```python
from build123d import *

# Parameters (mm, degrees)
SKETCH2_R               = 22.5
BOSS_EXTRUDE1_DEPTH     = 15
BOSS_EXTRUDE2_DEPTH     = 22
CUT_EXTRUDE2_DEPTH      = 119.676029593
CUT_EXTRUDE2_DEPTH_BACK = 119.676029593
FILLET1_R               = 100
CUT_EXTRUDE3_START      = -27.5
CUT_EXTRUDE3_DEPTH      = 4
CUT_EXTRUDE3_DRAFT      = -3
CUT_EXTRUDE7_DEPTH      = 183.208671748
CUT_EXTRUDE7_DEPTH_BACK = 183.208671748


with BuildPart() as part:
    # Sketch2 → Boss-Extrude1 (new body)
    with BuildSketch(Plane(origin=(0, 0, 0), x_dir=(0, 0, -1), z_dir=(1, 0, 0))):
        Circle(SKETCH2_R)
    extrude(amount=BOSS_EXTRUDE1_DEPTH)

    # Sketch3 → Boss-Extrude2 (add)
    with BuildSketch(Plane(origin=(0, 0, 0), x_dir=(0, 0, -1), z_dir=(1, 0, 0))):
        with BuildLine():
            Line((-27.5, 0), (-27.5, -20))
            Line((-27.5, -20), (-60, -40))
            ThreePointArc((-60, -40), (0, -100), (60, -40))
            Line((60, -40), (27.5, -20))
            Line((27.5, -20), (27.5, 0))
            ThreePointArc((27.5, 0), (0, 27.5), (-27.5, 0))
        make_face()
    extrude(amount=-BOSS_EXTRUDE2_DEPTH)

    # Sketch4 → Cut-Extrude2 (cut, two sides: drawn at the far end of the back side and taken through both)
    with BuildSketch(Plane.XY.offset(-CUT_EXTRUDE2_DEPTH_BACK)):
        Polygon((-12, 27.5), (-22, 27.5), (-22, -62.5), align=None)
    extrude(amount=CUT_EXTRUDE2_DEPTH + CUT_EXTRUDE2_DEPTH_BACK, mode=Mode.SUBTRACT)

    # Fillet1
    fillet1_edges = [part.edges().sort_by_distance(p)[0] for p in [
        (-22, -62.5, 0),
    ]]
    fillet(fillet1_edges, radius=FILLET1_R)

    # Sketch6 → Revolve1 (revolve)
    with BuildSketch(Plane.XY, mode=Mode.PRIVATE) as revolve1_sk:
        Polygon((-17, -17.5), (-45, -17.5), (-45, -25), (-60, -25), (-60, -27.5), (-110, -27.5), (-110, -40), (-17, -40), align=None)
    revolve(revolve1_sk.sketch.rotate(Axis((0, -40, 0), (1, 0, 0)), 90), axis=Axis((0, -40, 0), (1, 0, 0)))


with BuildPart() as cut_extrude3_tool:
    # Sketch8 → Cut-Extrude3 (with draft: the straight prism first)
    with BuildSketch(Plane(origin=(0, 0, 0), x_dir=(1, 0, 0), z_dir=(0, 1, 0)).offset(CUT_EXTRUDE3_START)):
        with BuildLine():
            ThreePointArc((-82, -4), (-78, 0), (-82, 4))
            Line((-82, 4), (-102, 4))
            ThreePointArc((-102, 4), (-106, 0), (-102, -4))
            Line((-102, -4), (-82, -4))
        make_face()
    extrude(amount=-CUT_EXTRUDE3_DEPTH)
    # Cut-Extrude3: the draft: its side faces are tilted about the plane it starts from
    cut_extrude3_sides = [cut_extrude3_tool.faces().sort_by_distance(p)[0] for p in [
        (-78, -29.5, 0),
        (-92, -29.5, -4),
        (-106, -29.5, 0),
        (-92, -29.5, 4),
    ]]
    draft(cut_extrude3_sides, Plane(origin=(0, 0, 0), x_dir=(1, 0, 0), z_dir=(0, 1, 0)).offset(CUT_EXTRUDE3_START), CUT_EXTRUDE3_DRAFT)


with BuildPart() as part_1:
    add(part.part)

    # Cut-Extrude3: cut by cut_extrude3_tool
    add(cut_extrude3_tool.part, mode=Mode.SUBTRACT)

    # Mirror2: part across plane


with BuildPart() as part_2:
    add(part_1.part)
    add(part_1.part.mirror(Plane(origin=(15, 0, 0), x_dir=(0, 0, 1), z_dir=(1, 0, 0))))

    # Sketch9 → Cut-Extrude7 (cut, two sides: drawn at the far end of the back side and taken through both)
    with BuildSketch(Plane.XY.offset(-CUT_EXTRUDE7_DEPTH_BACK)):
        Polygon((-60, -63.744180842), (-60, 19.972023277), (-60, 24.234333035), (-120.234198747, 24.234333035), (-120.234198747, -63.744180842), align=None)
    extrude(amount=CUT_EXTRUDE7_DEPTH + CUT_EXTRUDE7_DEPTH_BACK, mode=Mode.SUBTRACT)


solid = part_2.part
```
CAD build for the part. Positions are in the model's coordinates, mm. A direction names the side the tool comes from. Round coordinates to 2 decimals unless told otherwise and drop trailing zeros. Loops run counter-clockwise (first coordinate to the right, second up) from the corner with the lowest first, then second, coordinate; pieces in that order, holes last. Notation, with made-up numbers: M 5,37 L 57,37 A37 ccw 57,76 Z; hole C 0.5,10.25 d7. An arc over 180 degrees is marked long. Return JSON: item names as keys, results as strings. Group by question number.
(1) Saw through at D-D, the plane y = -50. List the corners of the cut face in (x, z).
(2) Tool access for faces 1 (the flat face through (-9, -10, 27.5)), 2 (the flat face through (-9, -10, -27.5)), 3 (the cylindrical face through (-31.196, -18.035, -4.878)): list every direction of +Z, -Z, +X, -X, +Y, -Y with a clear straight run to the whole face (end or side of a thin tool).
(3) Drop flat-ended pins along their axis: P1, Ø12, axis at y = -58, z = 32.5, coming from the +X side; P2, Ø16, axis at y = -83.5, z = -25, coming from the -X side; P3, Ø8, axis at x = -4.5, z = 46, coming from the -Y side. Give the stop position or say it passes through.
(4) Saw through at B-B, the plane x = -7.5. List the corners of the cut face in (y, z), and give its area (3 significant figures).
(5) Mould opens along X. For faces 4 (the conical face through (135.896, -29.472, -0.086)), 5 (the flat face through (39.61, -29.86, 43.52)), 6 (the flat face through (75, -35, 15)) say: +X half, -X half, draft (parallel to the pull), parting line (faces both ways), or undercut.
(6) Wall check: probe 1 along X at (y, z) = (-73, -39); probe 2 along X at (y, z) = (-29, -1); probe 3 along X at (y, z) = (0, -27). Give the ranges that are in metal, low to high. Write a range as [from, to].
(7) Saw through at A-A, the plane y = -88. List the corners of the cut face in (x, z), and give its area (3 significant figures).
Answer list:
{
 "1": {"outline": "M -60,-11.18 L -45,-11.18 L -45,-20.16 L -20.61,-20.16 L -20.61,-59.16 L 0,-59.16 L 0,59.16 L -20.61,59.16 L -20.61,20.16 L -45,20.16 L -45,11.18 L -60,11.18 Z; M 30,-59.16 L 50.61,-59.16 L 50.61,-20.16 L 75,-20.16 L 75,-11.18 L 90,-11.18 L 90,-7.5 L 140,-7.5 L 140,7.5 L 90,7.5 L 90,11.18 L 75,11.18 L 75,20.16 L 50.61,20.16 L 50.61,59.16 L 30,59.16 Z"},
 "2": {"face 1": "+Z, +X, -X, +Y", "face 2": "-Z, +X, -X, +Y", "face 3": "-X"},
 "3": {"P1": "x = 51.92", "P2": "x = -22", "P3": "y = -82.85"},
 "4": {"outline": "M -40,-60 L -20,-27.5 L 0,-27.5 A27.5 ccw 0,27.5 L -20,27.5 L -40,60 A60 ccw Z", "area": "9,690 mm2"},
 "5": {"face 4": "undercut", "face 5": "draft", "face 6": "+X half"},
 "6": {"probe 1": "[-22, 0], [30, 52]", "probe 2": "[-60, 0], [30, 108.21], [135.79, 140]", "probe 3": "[-15.06, 0], [30, 45.06]"},
 "7": {"outline": "M -22,-36 L 0,-36 L 0,36 L -22,36 Z; M 30,-36 L 52,-36 L 52,36 L 30,36 Z", "area": "3,170 mm2"}
}
